Check sheet for the modelled part. Datum: model origin and axes. Units: mm. Face numbers are marked on the shaded views. A direction names the side the tool comes from. Round coordinates to 2 decimals unless told otherwise and drop trailing zeros. Write each loop counter-clockwise with the first axis right and the second up, starting at its lowest first coordinate (ties: lowest second). Pieces come first, ordered by that corner, then holes. Notation, with made-up numbers: M -14,-3 L 42,-3 A20 cw 42,3 Z; hole C 22,-20.75 d5. An arc over 180 degrees is marked long. Put each result on its own line as item: value.
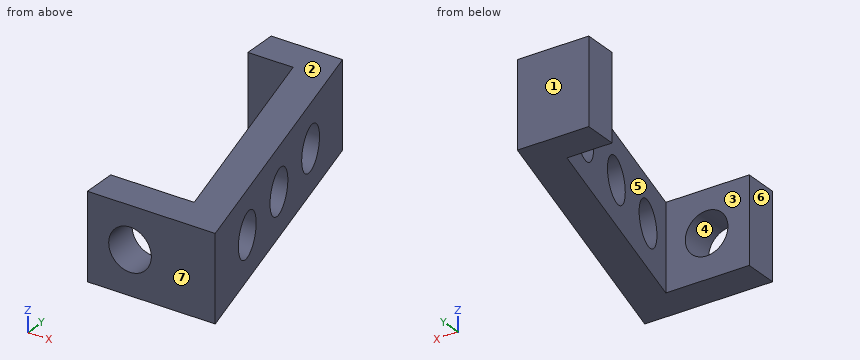
```python
from build123d import *

# Parameters (mm, degrees)
BOSS_EXTRUDE1_DEPTH     = 10
CUT_EXTRUDE1_DEPTH      = 10
CUT_EXTRUDE1_DEPTH_BACK = 15
SKETCH2_R               = 2.5
SKETCH3_R               = 2.5
CUT_EXTRUDE2_DEPTH      = 15


with BuildPart() as part:
    # Sketch1 → Boss-Extrude1 (new body)
    with BuildSketch(Plane.XY):
        Polygon((-6.068965517, -4), (8.931034483, -4), (-0.661546606, 31.8), (-9.036163723, 31.8), (-9.036163723, 27.802335145), (-3.731480258, 27.802335145), (3.718132991, 0), (-6.068965517, 0), align=None)
    extrude(amount=BOSS_EXTRUDE1_DEPTH)

    # Sketch2 → Cut-Extrude1 (cut, two sides: drawn at the far end of the back side and taken through both)
    with BuildSketch(Plane.ZY.offset(6.068965517).offset(-CUT_EXTRUDE1_DEPTH_BACK)):
        with Locations(Location((5, 22.802335145, 0), (0, 0, 270))):
            Circle(SKETCH2_R)
        with Locations(Location((5, 5, 0), (0, 0, 270))):
            Circle(SKETCH2_R)
        with Locations(Location((5, 13.9, 0), (0, 0, 270))):
            Circle(SKETCH2_R)
    extrude(amount=CUT_EXTRUDE1_DEPTH + CUT_EXTRUDE1_DEPTH_BACK, mode=Mode.SUBTRACT)

    # Sketch3 → Cut-Extrude2 (cut)
    with BuildSketch(Plane(origin=(0, 0, 0), x_dir=(1, 0, 0), z_dir=(0, 1, 0))):
        with Locations(Location((-1.068965517, -5.100482612, 0), (0, 0, 180))):
            Circle(SKETCH3_R)
    extrude(amount=-CUT_EXTRUDE2_DEPTH, mode=Mode.SUBTRACT)


solid = part.part
```
1. Cross-section at C-C (x = 0.25). Enter the section's corners in (y, z), then the cut area to 3 significant figures.
Computed values:
outline: M -4,0 L 0,0 L 0,2.98 L -4,2.98 Z; M -4,7.22 L 0,7.22 L 0,10 L -4,10 Z; M 12.94,0 L 28.4,0 L 28.4,10 L 12.94,10 L 12.94,7.31 A2.5 cw long 12.94,2.69 Z; hole C 22.8,5 d5
area: 143 mm2
2. Cross-section at A-A (y = 13.9). Enter the section's corners in (x, z).
Computed values:
outline: M -0.01,0 L 4.13,0 L 4.13,2.5 L -0.01,2.5 Z; M -0.01,7.5 L 4.13,7.5 L 4.13,10 L -0.01,10 Z
3. Scan lines: probe 1 along Z at (x, y) = (4, 5); probe 2 along Y at (x, z) = (-5.75, 5.25); probe 3 along Y at (x, z) = (-2.75, 5). Record each from-to range of solid material in increasing order.
Computed values:
probe 1: z = 0 to 2.5, 7.5 to 10
probe 2: y = -4 to 0, 27.8 to 31.8
probe 3: y = 25.3 to 31.8
4. Access from +Z, -Z, +X, -X, +Y, -Y to the whole of each face (thin tool, end or side, straight path). Record for the marked faces 4, 5, 6 and 7.
Computed values:
face 4: -Y
face 5: +Z, -Z, -X
face 6: +Z, -Z, -X, -Y
face 7: +Z, -Z, +X, -X, -Y
5. Depth check by flat-ended pin: pin 1 Ø4 at (y, z) = (7, 2.5) entering from -X; pin 2 Ø1 at (y, z) = (16, 3) entering from -X; pin 3 Ø1.2 at (y, z) = (-1, 7.5) entering from -X. Enter the tip coordinate at first touch or a pass-through.
Computed values:
pin 1: stops at x = 1.31
pin 2: stops at x = -0.7
pin 3: stops at x = -6.07
6. Cross-section at B-B (z = 0.75). Enter the section's corners in (x, y), then the cut area to 3 significant figures.
Computed values:
outline: M -9.04,27.8 L -3.73,27.8 L 3.72,0 L -6.07,0 L -6.07,-4 L 8.93,-4 L -0.66,31.8 L -9.04,31.8 Z
area: 209 mm2
7. Release check for a two-part mould opening along Y. For the marked faces 1, 2 and 3 record: +Y half, -Y half, draft (parallel to the pull), parting line (faces both ways), or undercut.
Computed values:
face 1: +Y half
face 2: draft
face 3: undercut
8. Cross-section at D-D (z = 3.75). Enter the section's corners in (x, y).
Computed values:
outline: M -9.04,27.8 L -3.73,27.8 L -2.97,24.97 L 1.17,24.97 L -0.66,31.8 L -9.04,31.8 Z; M -6.07,-4 L -3.17,-4 L -3.17,0 L -6.07,0 Z; M -1.81,20.64 L -0.59,16.07 L 3.55,16.07 L 2.33,20.64 Z; M 0.57,11.73 L 1.8,7.17 L 5.94,7.17 L 4.71,11.73 Z; M 1.03,-4 L 8.93,-4 L 7.1,2.83 L 2.96,2.83 L 3.72,0 L 1.03,0 Z
